from build123d import *

# Parameters (mm, degrees)
SKETCH_1_R          = 4.5
SKETCH_1_R_2        = 4
EXTRUDE_1_DEPTH     = 4.5
SKETCH_2_W          = 11
SKETCH_2_H          = 11
SKETCH_2_R          = 4
EXTRUDE_2_DEPTH     = 0.5
SKETCH_3_W          = 6.1
SKETCH_3_H          = 7.1
CUT_EXTRUDE_1_DEPTH = 0.2
SKETCH_4_W          = 11
SKETCH_4_H          = 11
SKETCH_4_W_2        = 10.05
SKETCH_4_H_2        = 10.05
EXTRUDE_3_DEPTH     = 1.2
SKETCH_5_R          = 0.5
EXTRUDE_4_DEPTH     = 1.25
SKETCH_6_R          = 1
SKETCH_6_R_2        = 0.5
EXTRUDE_5_DEPTH     = 0.75
EXTRUDE_5_2_DEPTH   = 0.75
EXTRUDE_6_DEPTH     = 0.7
FILLET_1_R          = 3
EXTRUDE_7_DEPTH     = 0.9
EXTRUDE_8_DEPTH     = 0.2
SKETCH_12_R         = 4.5
CUT_EXTRUDE_2_DEPTH = 0.001
SKETCH_13_R         = 4.0375
CUT_EXTRUDE_3_DEPTH = 4.799
SKETCH_20_R         = 1.5
EXTRUDE_10_DEPTH    = 1.8
SKETCH_21_R         = 0.875
CUT_EXTRUDE_5_DEPTH = 3


with BuildPart() as part:
    # Sketch 1 → Extrude 1 (new body)
    with BuildSketch(Plane(origin=(0, 0, 0), x_dir=(1, 0, 0), z_dir=(0, 1, 0))):
        with Locations(Location((0, 0, 0), (0, 0, 270))):
            Circle(SKETCH_1_R)
        with Locations(Location((0, 0, 0), (0, 0, 270))):
            Circle(SKETCH_1_R_2, mode=Mode.SUBTRACT)
    extrude(amount=EXTRUDE_1_DEPTH)

    # Sketch 2 → Extrude 2 (add)
    with BuildSketch(Plane(origin=(0, 4.5, 0), x_dir=(1, 0, 0), z_dir=(0, 1, 0))):
        Rectangle(SKETCH_2_W, SKETCH_2_H)
        with Locations(Location((0, 0, 0), (0, 0, 270))):
            Circle(SKETCH_2_R, mode=Mode.SUBTRACT)
    extrude(amount=EXTRUDE_2_DEPTH)

    # Sketch 3 → Cut-Extrude 1 (cut)
    with BuildSketch(Plane(origin=(0, 5, 0), x_dir=(1, 0, 0), z_dir=(0, 1, 0))):
        Rectangle(SKETCH_3_W, SKETCH_3_H)
    extrude(amount=-CUT_EXTRUDE_1_DEPTH, mode=Mode.SUBTRACT)

    # Sketch 4 → Extrude 3 (add)
    with BuildSketch(Plane(origin=(0, 5, 0), x_dir=(1, 0, 0), z_dir=(0, 1, 0))):
        Rectangle(SKETCH_4_W, SKETCH_4_H)
        Rectangle(SKETCH_4_W_2, SKETCH_4_H_2, mode=Mode.SUBTRACT)
    extrude(amount=EXTRUDE_3_DEPTH)

    # Sketch 5 → Extrude 4 (add)
    with BuildSketch(Plane(origin=(0, 6.2, 0), x_dir=(1, 0, 0), z_dir=(0, 1, 0))):
        with BuildLine():
            Line((5.5, 1), (5.5, -1))
            Line((5.5, -1), (6.6, -1))
            ThreePointArc((6.6, -1), (7.6, 0), (6.6, 1))
            Line((6.6, 1), (5.5, 1))
        make_face()
        with Locations(Location((6.6, 0, 0), (0, 0, 270))):
            Circle(SKETCH_5_R, mode=Mode.SUBTRACT)
        with BuildLine():
            Line((-6.6, -1), (-5.5, -1))
            Line((-5.5, -1), (-5.5, 1))
            Line((-5.5, 1), (-6.6, 1))
            ThreePointArc((-6.6, 1), (-7.6, 0), (-6.6, -1))
        make_face()
        with Locations(Location((-6.6, 0, 0), (0, 0, 270))):
            Circle(SKETCH_5_R, mode=Mode.SUBTRACT)
    extrude(amount=-EXTRUDE_4_DEPTH)



with BuildPart() as body_2:
    # Sketch 6 → Extrude 5 (new, symmetric)
    with BuildSketch(Plane.XY.offset(5.5)):
        with Locations((-6.6, -0.8)):
            Circle(SKETCH_6_R)
        with Locations((-6.6, -0.8)):
            Circle(SKETCH_6_R_2, mode=Mode.SUBTRACT)
    extrude(amount=EXTRUDE_5_DEPTH, both=True)



with BuildPart() as body_3:
    # Sketch 6 → Extrude 5 2 (new, symmetric)
    with BuildSketch(Plane.XY.offset(5.5)):
        with Locations(Location((6.6, -0.8, 0), (0, 0, 180))):
            Circle(SKETCH_6_R)
        with Locations(Location((6.6, -0.8, 0), (0, 0, 180))):
            Circle(SKETCH_6_R_2, mode=Mode.SUBTRACT)
    extrude(amount=EXTRUDE_5_2_DEPTH, both=True)


with BuildPart() as body_2_1:
    add(body_2.part)

    add(body_3.part)  # Extrude 6 merges body 3
    # Sketch 7 → Extrude 6 (add, symmetric)
    with BuildSketch(Plane.XY.offset(5.5)):
        Polygon((-6.469610026, 0.091907201), (0, 3.160138746), (6.469610026, 0.091907201), (5.826851035, -1.263401207), (0, 1.5), (-5.826851035, -1.263401207), align=None)
    extrude(amount=EXTRUDE_6_DEPTH, both=True)

    # Fillet 1
    fillet_1_edges = [body_2_1.edges().sort_by_distance(p)[0] for p in [
        (0, 1.5, 5.5),
        (0, 3.160138746, 5.5),
    ]]
    fillet(fillet_1_edges, radius=FILLET_1_R)


with BuildPart() as part_1:
    add(part.part)

    add(body_2_1.part)  # Extrude 7 merges body 2
    # Sketch 8 → Extrude 7 (add)
    with BuildSketch(Plane(origin=(0, 0, 4.8), x_dir=(-1, 0, 0), z_dir=(0, 0, -1))):
        with BuildLine():
            Line((1.5, 2.448759343), (1.5, 0.788620597))
            Line((1.5, 0.788620597), (1.285517981, 0.890339324))
            ThreePointArc((1.285517981, 0.890339324), (0, 1.179722509), (-1.285517981, 0.890339324))
            Line((-1.285517981, 0.890339324), (-1.5, 0.788620597))
            Line((-1.5, 0.788620597), (-1.5, 2.448759343))
            Line((-1.5, 2.448759343), (-1.285517981, 2.55047807))
            ThreePointArc((-1.285517981, 2.55047807), (0, 2.839861254), (1.285517981, 2.55047807))
            Line((1.285517981, 2.55047807), (1.5, 2.448759343))
        make_face()
    extrude(amount=EXTRUDE_7_DEPTH)

    # Sketch 11 → Extrude 8 (add)
    with BuildSketch(Plane(origin=(0, 5, 0), x_dir=(1, 0, 0), z_dir=(0, 1, 0))):
        with BuildLine():
            Line((-3.05, 2.587952859), (-3.05, -2.587952859))
            ThreePointArc((-3.05, -2.587952859), (-4, 0), (-3.05, 2.587952859))
        make_face()
        with BuildLine():
            Line((3.05, 2.587952859), (3.05, -2.587952859))
            ThreePointArc((3.05, -2.587952859), (4, 0), (3.05, 2.587952859))
        make_face()
        with BuildLine():
            Line((-1.843230859, 3.55), (1.843230859, 3.55))
            ThreePointArc((1.843230859, 3.55), (0, 4), (-1.843230859, 3.55))
        make_face()
        with BuildLine():
            Line((-1.843230859, -3.55), (1.843230859, -3.55))
            ThreePointArc((1.843230859, -3.55), (0, -4), (-1.843230859, -3.55))
        make_face()
    extrude(amount=-EXTRUDE_8_DEPTH)

    # Sketch 12 → Cut-Extrude 2 (cut)
    with BuildSketch(Plane.XZ):
        with Locations(Location((0, 0, 0), (0, 0, 270))):
            Circle(SKETCH_12_R)
    extrude(amount=-CUT_EXTRUDE_2_DEPTH, mode=Mode.SUBTRACT)

    # Sketch 13 → Cut-Extrude 3 (cut)
    with BuildSketch(Plane.XZ.offset(-0.001)):
        with Locations(Location((0, 0, 0), (0, 0, 270))):
            Circle(SKETCH_13_R)
    extrude(amount=-CUT_EXTRUDE_3_DEPTH, mode=Mode.SUBTRACT)

    # Sketch 20 → Extrude 10 (add)
    with BuildSketch(Plane.ZY.offset(6)):
        with Locations((0, 2.657828557)):
            Circle(SKETCH_20_R)
    extrude_10 = extrude(amount=-EXTRUDE_10_DEPTH)

    # Sketch 21 → Cut-Extrude 5 (cut)
    with BuildSketch(Plane.ZY.offset(6)):
        with Locations((0, 2.657828557)):
            Circle(SKETCH_21_R)
    cut_extrude_5 = extrude(amount=-CUT_EXTRUDE_5_DEPTH, mode=Mode.SUBTRACT)

    # Mirror 3: Extrude 10, Cut-Extrude 5 across plane
    add(extrude_10.mirror(Plane(origin=(0, 0, 0), x_dir=(0, 0, 1), z_dir=(1, 0, 0))))
    add(cut_extrude_5.mirror(Plane(origin=(0, 0, 0), x_dir=(0, 0, 1), z_dir=(1, 0, 0))), mode=Mode.SUBTRACT)


solid = part_1.part
Source: CAD feature listing. Evaluate the final solid. Frame: model axes, mm. A direction names the side the tool comes from. Give positions to 0.01 mm unless a question says otherwise; leave off trailing zeros. Write each loop counter-clockwise with the first axis right and the second up, starting at its lowest first coordinate (ties: lowest second). Pieces come first, ordered by that corner, then holes. Notation, with made-up numbers: M 52,-6.5 L 97,-6.5 A36 cw 97,31.5 Z; hole C 77,3 d11. An arc over 180 degrees is marked long. Return JSON: item names as keys, results as strings. Group by question number.
1) Set-up query: faces 5 (the face through (-2.7, 4.8, -3.3)), 6 (the face through (0, 5, 5.5)), 7 (the face through (-0.02, 1.18, 5.27)), 8 (the face through (0, 5, -5.5)). Return all of +Z, -Z, +X, -X, +Y, -Y with unobstructed straight access to the full face (end or side cutting, diameter ignored); none if empty.
2) Cut plane C-C, the plane z = 0. Give the number of separate pieces and of enclosed holes in the cut face, plus the area to 3 significant figures.
3) Material intervals for line 1 along X through (y, z) = (5.55, 0) (3 decimals); line 2 along Y through (x, z) = (-6.6, 5.9); line 3 along Z through (x, y) = (-0.5, 5.5) (3 decimals), sorted ascending. Write a range as [from, to].
4) Cut plane D-D, the plane x = -2.75. Output: boundary loops of the cut face in (y, z) (3 decimals).
5) Pin query (flat end, axial travel): P1, Ø1, axis at x = -6.5, y = -0.5, coming from the -Z side; P2, Ø4, axis at x = -5, y = 1, coming from the -Z side; P3, Ø2, axis at x = 0, y = 0, coming from the +Z side; P4, Ø1.4, axis at y = 2.66, z = 0, coming from the -X side. Return the tip coordinate at first contact, or that it passes through.
6) Pull-direction query (X, two-part tool) for faces 1 (the face through (-3.4, 4.8, 0)), 2 (the face through (6, 6, 1)), 3 (the face through (-7.4, -1.4, 5.5)), 4 (the face through (0.02, 2.84, 5.27)); classes: pulls with the +X half, pulls with the -X half, needs draft (parallel to the pull), parting line crosses it, or undercut.
7) Cut plane B-B, the plane y = -0.8. Output: boundary loops of the cut face in (x, z), plus the area to 3 significant figures.
Recorded:
{
 "1": {"face 5": "+Y", "face 6": "+Z, +X, -X, +Y", "face 7": "+Z, -Y", "face 8": "-Z, +X, -X, +Y, -Y"},
 "2": {"separate pieces": "6", "enclosed holes": "0", "area": "12.0 mm²"},
 "3": {"line 1": "x = [-7.6, -7.1], [-6.1, -5.025], [5.025, 6.1], [7.1, 7.6]", "line 2": "y = [-1.8, -1.3], [-0.3, 0.2]", "line 3": "z = [-5.5, -5.025], [5.025, 5.5]"},
 "4": {"outline": "M 0.001,-3.562 L 4.5,-3.562 L 4.5,-5.5 L 6.2,-5.5 L 6.2,-5.025 L 5,-5.025 L 5,-3.55 L 4.8,-3.55 L 4.8,-2.956 L 0.001,-2.956 Z; M 0.001,2.956 L 4.8,2.956 L 4.8,3.55 L 5,3.55 L 5,5.025 L 6.2,5.025 L 6.2,5.5 L 4.5,5.5 L 4.5,3.562 L 0.001,3.562 Z; M 0.196,4.8 L 1.856,4.8 L 1.856,6.2 L 0.196,6.2 Z"},
 "5": {"P1": "stops at z = 4.75", "P2": "stops at z = -3.35", "P3": "stops at z = 4.5", "P4": "passes through"},
 "6": {"face 1": "undercut", "face 2": "needs draft", "face 3": "undercut", "face 4": "parting line crosses it"},
 "7": {"outline": "M -7.6,4.75 L -7.1,4.75 L -7.1,6.25 L -7.6,6.25 Z; M -6.1,4.75 L -5.6,4.75 L -5.6,4.8 L -4.85,4.8 L -4.85,6.2 L -5.6,6.2 L -5.6,6.25 L -6.1,6.25 Z; M 4.85,4.8 L 5.6,4.8 L 5.6,4.75 L 6.1,4.75 L 6.1,6.25 L 5.6,6.25 L 5.6,6.2 L 4.85,6.2 Z; M 7.1,4.75 L 7.6,4.75 L 7.6,6.25 L 7.1,6.25 Z", "area": "5.10 mm²"}
}
